Design review of the part built by this model. Coordinates are the model's own, in mm. A direction names the side the tool comes from. Round coordinates to 2 decimals unless told otherwise and drop trailing zeros. Loops run counter-clockwise (first coordinate to the right, second up) from the corner with the lowest first, then second, coordinate; pieces in that order, holes last. Notation, with made-up numbers: (-35, 19.5) -> (-25, 19.5) arc R19 ccw to (-25, 35.5) -> close; hole circle Ø3 at (-11, -29). An arc over 180 degrees is marked (long way). Answer as CSV lines item,"result". Start each with the question number.
(1) Take a section at B-B, the plane z = -22.5. Write out the cut boundary in (x, y), and give its area (3 significant figures).
(2) Take a section at D-D, the plane x = -78. Write out the cut boundary in (y, z).
(3) Draft analysis for pull direction X (two halves, no side actions). For faces 1 (the face through (-101.5, 795, -59)), 2 (the face through (-81.5, 795.209, -23.357)), 3 (the face through (82.266, 795.209, -22.714)), state which applies: +X half, -X half, draft (parallel to the pull), parting line (faces both ways), or undercut.
(4) To check wall thickness, follow line 1 (Y direction, x = 101, z = -60); line 2 (X direction, y = 1192, z = -59.5); line 3 (X direction, y = 941, z = -22). State the ranges of each line that lie inside material, in increasing order. Write a range as from..to.
(5) Take a section at A-A, the plane y = 341.5. Write out the cut boundary in (x, z), and give its area (3 significant figures).
(6) For P1, Ø10.5, axis at y = 542, z = -60.5, coming from the +X side; P2, Ø2, axis at x = 20.5, y = 900.5, coming from the -Z side; P3, Ø10, axis at x = -74.5, y = 402, coming from the +Z side; P4, Ø10, axis at x = -7, z = -7.5, coming from the +Y side, all flat-tipped, find the tip position at first contact; note any pin that passes through.
(7) Take a section at C-C, the plane x = -10. Write out the cut boundary in (y, z), and give its area (3 significant figures).
(8) Machinability: for faces 4 (the face through (1, 795, 1)), 5 (the face through (-100.5, 795, -60)), which of the approach directions +Z, -Z, +X, -X, +Y, -Y give a long, thin tool a straight path to every point of the face, cutting with its end or side? Answer none if there is none.
from build123d import *

# Parameters (mm, degrees)
BASE_FLANGE1_DEPTH = 1613
FILLET1_R          = 3
CUT_EXTRUDE4_REACH = 1629.362
SKETCH10_R         = 3.25
LPATTERN5_COUNT    = 4
LPATTERN5_PITCH    = 529


# Sheet-metal steps are written as plain solids
with BuildPart() as part:
    # Sketch1 → Base-Flange1 (new body)
    with BuildSketch(Plane(origin=(0, 0, 0), x_dir=(1, 0, 0), z_dir=(0, 1, 0))):
        with BuildLine():
            Line((-100.5, 73), (-100.5, 46.363970234))
            ThreePointArc((-100.5, 46.363970234), (-100.439692621, 46.021950091), (-100.266044443, 45.721182625))
            Line((-100.266044443, 45.721182625), (-62.201153751, 0.35721239))
            ThreePointArc((-62.201153751, 0.35721239), (-61.857727569, 0.093692213), (-61.435109308, 0))
            Line((-61.435109308, 0), (61.435109308, 0))
            ThreePointArc((61.435109308, 0), (61.857727569, 0.093692213), (62.201153751, 0.35721239))
            Line((62.201153751, 0.35721239), (100.266044443, 45.721182625))
            ThreePointArc((100.266044443, 45.721182625), (100.439692621, 46.021950091), (100.5, 46.363970234))
            Line((100.5, 46.363970234), (100.5, 73))
            Line((100.5, 73), (101.5, 73))
            Line((101.5, 73), (101.5, 46.363970234))
            ThreePointArc((101.5, 46.363970234), (101.379385242, 45.679929948), (101.032088886, 45.078395015))
            Line((101.032088886, 45.078395015), (62.967198194, -0.285575219))
            ThreePointArc((62.967198194, -0.285575219), (62.280345831, -0.812615574), (61.435109308, -1))
            Line((61.435109308, -1), (-61.435109308, -1))
            ThreePointArc((-61.435109308, -1), (-62.280345831, -0.812615574), (-62.967198194, -0.285575219))
            Line((-62.967198194, -0.285575219), (-101.032088886, 45.078395015))
            ThreePointArc((-101.032088886, 45.078395015), (-101.379385242, 45.679929948), (-101.5, 46.363970234))
            Line((-101.5, 46.363970234), (-101.5, 73))
            Line((-101.5, 73), (-100.5, 73))
        make_face()
    extrude(amount=BASE_FLANGE1_DEPTH)

    # Fillet1
    fillet1_edges = [part.edges().sort_by_distance(p)[0] for p in [
        (-101, 0, -73),
        (101, 0, -73),
        (-101, 1613, -73),
        (101, 1613, -73),
    ]]
    fillet(fillet1_edges, radius=FILLET1_R)

    # Cut-Extrude4: up to this face of the body (flat: up to its plane)
    cut_extrude4_end = Plane(part.part.faces().sort_by_distance((-101.5, 806.5, -59.680847857))[0])
    # Sketch10 → Cut-Extrude4 (cut, up to the picked face)
    with BuildSketch(Plane(origin=(101.5, 0, 0), x_dir=(0, 0, -1), z_dir=(1, 0, 0)), mode=Mode.PRIVATE) as cut_extrude4_sk1:
        with Locations((60.5, 13)):
            Circle(SKETCH10_R)
    cut_extrude4_tool1 = split(extrude(cut_extrude4_sk1.sketch, amount=-CUT_EXTRUDE4_REACH, mode=Mode.PRIVATE), bisect_by=cut_extrude4_end, keep=Keep.BOTH, mode=Mode.PRIVATE)
    cut_extrude4 = cut_extrude4_tool1.solids().sort_by(Axis((101.5, 13, -60.5), (-1, 0, 0)))[0]
    add(cut_extrude4, mode=Mode.SUBTRACT)

    # LPattern5: Cut-Extrude4 ×4
    with Locations(*[(0, i * LPATTERN5_PITCH, 0) for i in range(1, LPATTERN5_COUNT)]):
        add(cut_extrude4, mode=Mode.SUBTRACT)


solid = part.part
The answers:
1,outline,"(-82.09, 0) -> (-80.78, 0) -> (-80.78, 1613) -> (-82.09, 1613) -> close; (80.78, 0) -> (82.09, 0) -> (82.09, 1613) -> (80.78, 1613) -> close"
1,area,"4,210 mm²"
2,outline,"(0, -19.19) -> (1613, -19.19) -> (1613, -17.63) -> (0, -17.63) -> close"
3,face 1,"-X half"
3,face 2,"undercut"
3,face 3,"+X half"
4,line 1,"0..9.79, 16.21..538.79, 545.21..1067.79, 1074.21..1596.79, 1603.21..1613"
4,line 2,"-101.5..-100.5, 100.5..101.5"
4,line 3,"-81.67..-80.36, 80.36..81.67"
5,outline,"(-101.5, -73) -> (-100.5, -73) -> (-100.5, -46.36) arc R1 cw to (-100.27, -45.72) -> (-62.2, -0.36) arc R1 cw to (-61.44, 0) -> (61.44, 0) arc R1 cw to (62.2, -0.36) -> (100.27, -45.72) arc R1 cw to (100.5, -46.36) -> (100.5, -73) -> (101.5, -73) -> (101.5, -46.36) arc R2 ccw to (101.03, -45.08) -> (62.97, 0.29) arc R2 ccw to (61.44, 1) -> (-61.44, 1) arc R2 ccw to (-62.97, 0.29) -> (-101.03, -45.08) arc R2 ccw to (-101.5, -46.36) -> close"
5,area,"299 mm²"
6,P1,"x = 101.5"
6,P2,"z = 0"
6,P3,"z = -7.5"
6,P4,"through"
7,outline,"(0, 0) -> (1613, 0) -> (1613, 1) -> (0, 1) -> close"
7,area,"1,610 mm²"
8,face 4,"+Z, +X, -X, +Y, -Y"
8,face 5,"-Z, +Y, -Y"
